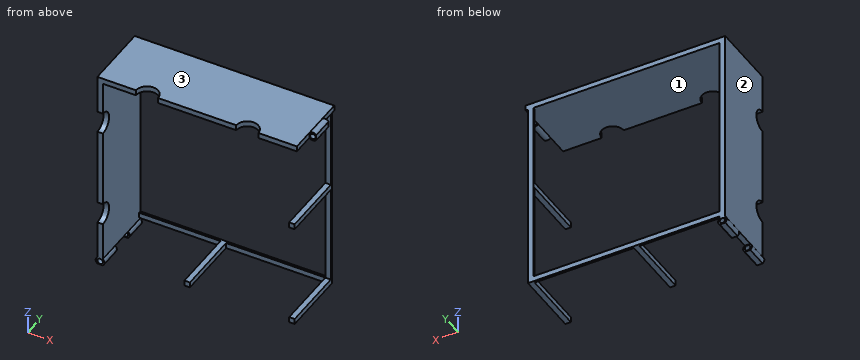
```python
from build123d import *

# Parameters (mm, degrees)
BOSS_EXTRUDE1_DEPTH     = 60
SKETCH2_R               = 2.5
CUT_EXTRUDE1_DEPTH      = 60
SKETCH4_W               = 7.122498999
SKETCH4_H               = 20
CUT_EXTRUDE3_DEPTH      = 2.5
CUT_EXTRUDE3_DEPTH_BACK = 189
CUT_EXTRUDE4_DEPTH      = 21
CUT_EXTRUDE4_DEPTH_BACK = 41
SKETCH6_W               = 8.505604829
SKETCH6_H               = 20.5
CUT_EXTRUDE6_DEPTH      = 2.5
CUT_EXTRUDE6_DEPTH_BACK = 188.122498999
CUT_EXTRUDE7_DEPTH      = 1
CUT_EXTRUDE7_DEPTH_BACK = 61
BOSS_EXTRUDE2_DEPTH     = 2
SKETCH9_W               = 5
SKETCH9_H               = 5
BOSS_EXTRUDE3_DEPTH     = 58


with BuildPart() as part:
    # Sketch1 → Boss-Extrude1 (new body)
    with BuildSketch(Plane(origin=(0, 0, 0), x_dir=(1, 0, 0), z_dir=(0, 1, 0))):
        with BuildLine():
            Line((0, 0), (180, 0))
            Line((180, 0), (180.877501001, 0))
            ThreePointArc((180.877501001, 0), (188, 2.5), (180.877501001, 5))
            Line((180.877501001, 5), (180, 5))
            Line((180, 5), (5, 5))
            Line((5, 5), (5, 180))
            Line((5, 180), (5, 180.877501001))
            ThreePointArc((5, 180.877501001), (2.5, 188), (0, 180.877501001))
            Line((0, 180.877501001), (0, 180))
            Line((0, 180), (0, 0))
        make_face()
    extrude(amount=BOSS_EXTRUDE1_DEPTH)

    # Sketch2 → Cut-Extrude1 (cut)
    with BuildSketch(Plane(origin=(0, 60, 0), x_dir=(1, 0, 0), z_dir=(0, 1, 0))):
        with Locations((184, 2.5)):
            Circle(SKETCH2_R)
        with Locations((2.5, 184)):
            Circle(SKETCH2_R)
    extrude(amount=-CUT_EXTRUDE1_DEPTH, mode=Mode.SUBTRACT)

    # Sketch4 → Cut-Extrude3 (cut, two sides)
    with BuildSketch(Plane.XY) as cut_extrude3_sk:
        with BuildLine():
            ThreePointArc((35, 0), (45, -10), (55, 0))
            Line((55, 0), (45, 0))
            Line((45, 0), (35, 0))
        make_face()
        with BuildLine():
            Line((45, 0), (55, 0))
            ThreePointArc((55, 0), (45, 10), (35, 0))
            Line((35, 0), (45, 0))
        make_face()
        with BuildLine():
            ThreePointArc((125.877501001, 0), (135.877501001, -10), (145.877501001, 0))
            Line((145.877501001, 0), (135.877501001, 0))
            Line((135.877501001, 0), (125.877501001, 0))
        make_face()
        with BuildLine():
            Line((135.877501001, 0), (145.877501001, 0))
            ThreePointArc((145.877501001, 0), (135.877501001, 10), (125.877501001, 0))
            Line((125.877501001, 0), (135.877501001, 0))
        make_face()
        with Locations((184.438750501, 10)):
            Rectangle(SKETCH4_W, SKETCH4_H)
        with Locations((184.438750501, 50)):
            Rectangle(SKETCH4_W, SKETCH4_H)
    extrude(amount=CUT_EXTRUDE3_DEPTH, mode=Mode.SUBTRACT)
    extrude(cut_extrude3_sk.sketch, amount=-CUT_EXTRUDE3_DEPTH_BACK, mode=Mode.SUBTRACT)

    # Sketch5 → Cut-Extrude4 (cut, two sides)
    with BuildSketch(Plane(origin=(0, 40, 0), x_dir=(1, 0, 0), z_dir=(0, 1, 0))) as cut_extrude4_sk:
        with BuildLine():
            Line((187.122498999, 5), (187.122498999, 2.5))
            Line((187.122498999, 2.5), (187.122498999, 0))
            ThreePointArc((187.122498999, 0), (188, 2.5), (187.122498999, 5))
        make_face()
    extrude(amount=CUT_EXTRUDE4_DEPTH, mode=Mode.SUBTRACT)
    extrude(cut_extrude4_sk.sketch, amount=-CUT_EXTRUDE4_DEPTH_BACK, mode=Mode.SUBTRACT)

    # Sketch6 → Cut-Extrude6 (cut, two sides)
    with BuildSketch(Plane.ZY) as cut_extrude6_sk:
        with BuildLine():
            ThreePointArc((-145.877501001, 0), (-135.877501001, -10), (-125.877501001, 0))
            Line((-125.877501001, 0), (-135.877501001, 0))
            Line((-135.877501001, 0), (-145.877501001, 0))
        make_face()
        with BuildLine():
            Line((-135.877501001, 0), (-125.877501001, 0))
            ThreePointArc((-125.877501001, 0), (-135.877501001, 10), (-145.877501001, 0))
            Line((-145.877501001, 0), (-135.877501001, 0))
        make_face()
        with BuildLine():
            ThreePointArc((-55, 0), (-45, -10), (-35, 0))
            Line((-35, 0), (-45, 0))
            Line((-45, 0), (-55, 0))
        make_face()
        with BuildLine():
            Line((-45, 0), (-35, 0))
            ThreePointArc((-35, 0), (-45, 10), (-55, 0))
            Line((-55, 0), (-45, 0))
        make_face()
        with Locations((-185.130303416, 30)):
            Rectangle(SKETCH6_W, SKETCH6_H)
    extrude(amount=CUT_EXTRUDE6_DEPTH, mode=Mode.SUBTRACT)
    extrude(cut_extrude6_sk.sketch, amount=-CUT_EXTRUDE6_DEPTH_BACK, mode=Mode.SUBTRACT)

    # Sketch7 → Cut-Extrude7 (cut, two sides)
    with BuildSketch(Plane(origin=(0, 60, 0), x_dir=(1, 0, 0), z_dir=(0, 1, 0))) as cut_extrude7_sk:
        with BuildLine():
            ThreePointArc((5, 187.122498999), (2.5, 188), (0, 187.122498999))
            Line((0, 187.122498999), (2.5, 187.122498999))
            Line((2.5, 187.122498999), (5, 187.122498999))
        make_face()
    extrude(amount=CUT_EXTRUDE7_DEPTH, mode=Mode.SUBTRACT)
    extrude(cut_extrude7_sk.sketch, amount=-CUT_EXTRUDE7_DEPTH_BACK, mode=Mode.SUBTRACT)

    # Sketch8 → Boss-Extrude2 (add)
    with BuildSketch(Plane(origin=(0, 60, 0), x_dir=(1, 0, 0), z_dir=(0, 1, 0))):
        Polygon((178.877501001, 178.877501001), (5, 178.877501001), (5, 173.877501001), (173.877501001, 173.877501001), (173.877501001, 5), (178.877501001, 5), align=None)
    extrude(amount=-BOSS_EXTRUDE2_DEPTH)

    # Sketch9 → Boss-Extrude3 (add)
    with BuildSketch(Plane(origin=(0, 58, 0), x_dir=(-1, 0, 0), z_dir=(0, -1, 0))):
        with Locations((-176.377501001, 176.377501001)):
            Rectangle(SKETCH9_W, SKETCH9_H)
        with Locations((-176.377501001, 81.377501001)):
            Rectangle(SKETCH9_W, SKETCH9_H)
        with Locations((-81.377501001, 176.377501001)):
            Rectangle(SKETCH9_W, SKETCH9_H)
    extrude(amount=BOSS_EXTRUDE3_DEPTH)


solid = part.part
```
Part model, mm, in its own coordinate system. Face numbers are marked on the shaded views. Give positions to 0.01 mm unless a question says otherwise; leave off trailing zeros. Order: outer loops, then holes, each group sorted by start corner. A loop starts at its lowest first (then second) coordinate and runs counter-clockwise, first axis right, second up. Notation, with made-up numbers: (24, 46) - (59, 46) arc R18 ccw to (59, 61) - close; hole circle Ø8 at (35, 29). An arc over 180 degrees is marked (long way). Use one line per item in the form item = value.
Item 1: Slice it at D-D on z = -184. Give the cut face in (x, y), and give its area (4 significant figures).
Solution:
outline = (-1.5, 0) - (0, 0) - (0, 19.75) - (-1.5, 19.75) - close; (-1.5, 40.25) - (0, 40.25) - (0, 60) - (-1.5, 60) - close; (5, 0) - (6.5, 0) - (6.5, 19.75) - (5, 19.75) - close; (5, 40.25) - (6.5, 40.25) - (6.5, 60) - (5, 60) - close
area = 118.5 mm2
Item 2: Probe probe 1 along X at (y, z) = (29.25, -2.5); probe 2 along X at (y, z) = (7, -184); probe 3 along Z at (x, y) = (2.5, 53.5). List the from-to ranges inside material, lowest first. Write a range as from..to.
Solution:
probe_1 = 0..181.5, 186.5..187.12
probe_2 = -1.5..0, 5..6.5
probe_3 = -187.12..-186.5, -181.5..0
Item 3: Slice it at B-B on y = 44.5. Give the cut face in (x, z).
Solution:
outline = (0, -187.12) - (5, -187.12) arc R4 ccw to (5, -180.88) - (5, -5) - (180.88, -5) - (180.88, 0) - (0, 0) - (0, -180.88) arc R4 ccw to start; (78.88, -178.88) - (83.88, -178.88) - (83.88, -173.88) - (78.88, -173.88) - close; (173.88, -178.88) - (178.88, -178.88) - (178.88, -173.88) - (173.88, -173.88) - close; (173.88, -83.88) - (178.88, -83.88) - (178.88, -78.88) - (173.88, -78.88) - close; hole circle Ø5 at (2.5, -184)
Item 4: Slice it at C-C on x = 2.5. Give the cut face in (y, z).
Solution:
outline = (0, -187.12) - (19.75, -187.12) - (19.75, -186.5) - (0, -186.5) - close; (0, -181.5) - (19.75, -181.5) - (19.75, -180.88) - (40.25, -180.88) - (40.25, -181.5) - (60, -181.5) - (60, 0) - (0, 0) - (0, -35) arc R10 cw to (0, -55) - (0, -125.88) arc R10 cw to (0, -145.88) - close; (40.25, -187.12) - (60, -187.12) - (60, -186.5) - (40.25, -186.5) - close
Item 5: Slice it at A-A on z = -45. Give the cut face in (x, y).
Solution:
outline = (0, 10) - (5, 10) - (5, 60) - (0, 60) - close; (173.88, 58) - (178.88, 58) - (178.88, 60) - (173.88, 60) - close
Item 6: Pin check, flat tips, straight feed: pin 1 Ø5.5 at (x, z) = (53, -176) entering from -Y; pin 2 Ø4.5 at (x, z) = (2.5, -184) entering from -Y; pin 3 Ø1 at (x, y) = (155, 25.5) entering from +Z; pin 4 Ø1.5 at (y, z) = (22.5, -177.5) entering from -X. Stop position of each tip, or through.
Solution:
pin_1 = 58
pin_2 = through
pin_3 = 0
pin_4 = 0
Item 7: Two-plate mould, pull along X, no slides. Class the marked faces 1, 2 and 3: released by +X, released by -X, zero draft, split by the parting line, or undercut.
Solution:
face_1 = undercut
face_2 = released by -X
face_3 = zero draft
